from build123d import *

# Parameters (mm, degrees)
EXTRU_MINCE1_DEPTH    = 55
D_GAGEMENT_M41_D      = 4.5
D_GAGEMENT_M42_D      = 4.5
D_GAGEMENT_M271_D     = 30
D_GAGEMENT_M271_DEPTH = 1.5
D_GAGEMENT_M271_TIP   = 9.012909285


with BuildPart() as part:
    # Esquisse1 → Extru.-Mince1 (new body)
    with BuildSketch(Plane.XY):
        Polygon((0, 40), (0, 0), (25, 0), (25, 1.5), (1.5, 1.5), (1.5, 40), align=None)
    extrude(amount=-EXTRU_MINCE1_DEPTH)

    # Dégagement M41 (through all)
    with Locations(Plane(origin=(0, 1.5, 0), x_dir=(-1, 0, 0), z_dir=(0, 1, 0))):
        with Locations((-12.5, -7), (-12.5, -27.5), (-12.5, -48)):
            Hole(D_GAGEMENT_M41_D / 2)

    # Dégagement M42 (through all)
    with Locations(Plane(origin=(1.5, 0, 0), x_dir=(0, 0, -1), z_dir=(1, 0, 0))):
        with Locations((5, 34), (33, 6)):
            Hole(D_GAGEMENT_M42_D / 2)

    # Dégagement M271
    with Locations(Plane(origin=(1.5, 0, 0), x_dir=(0, 0, -1), z_dir=(1, 0, 0))):
        with Locations((19, 20)):
            Hole(D_GAGEMENT_M271_D / 2, depth=D_GAGEMENT_M271_DEPTH)
            with Locations((0, 0, -(D_GAGEMENT_M271_DEPTH + D_GAGEMENT_M271_TIP / 2))):  # 118° drill point
                Cone(0, D_GAGEMENT_M271_D / 2, D_GAGEMENT_M271_TIP, mode=Mode.SUBTRACT)


solid = part.part
Work out the finished part from the listing and answer in its coordinate system (mm). A direction names the side the tool comes from. Round coordinates to 2 decimals unless told otherwise and drop trailing zeros. Write each loop counter-clockwise with the first axis right and the second up, starting at its lowest first coordinate (ties: lowest second). Pieces come first, ordered by that corner, then holes.
1) The mould has two halves that part along Y. Classify faces 1 (the cylindrical face through (0.74, 6.676, -30.854)), 2 (the cylindrical face through (10.84, 0.74, -5.48)), 3 (the flat face through (10, 0, -27)): pulls with the +Y half, pulls with the -Y half, needs draft (parallel to the pull), parting line crosses it, or undercut.
2) A cutting plane is placed at B-B (z = -19). Give the vertices of the cut face in (x, y).
3) A cutting plane is placed at A-A (x = 12.5). Give the vertices of the cut face in (y, z), plus the area to 4 significant figures.
4) Straight lines are drawn through the part: line 1 (Z direction, x = 12.5, y = 0.35); line 2 (Z direction, x = 0.6, y = 20); line 3 (Y direction, x = 14.5, z = -37). For each, find the intervals that lie inside material, in ascending order.
5) A cutting plane is placed at D-D (z = -33). Give the vertices of the cut face in (x, y), plus the area to 3 significant figures.
6) Given pin 1 Ø1.5 at (x, z) = (11, -21) entering from -Y; pin 2 Ø11.5 at (y, z) = (12, -41) entering from +X, each flat-ended and moving along its own axis, determine where each tip first touches the part or whether it passes through.
7) A tool of negligible diameter and unlimited length cuts with its end or side. For faces 4 (the flat face through (16, 1.5, -27)), 5 (the cylindrical face through (0.74, 36.23, -5.29)), from which of +Z, -Z, +X, -X, +Y, -Y can it reach the whole face along a straight path? Write none if from no direction.
8) A cutting plane is placed at C-C (y = 34). Give the vertices of the cut face in (x, z).
Completed:
1. face 1: undercut
1. face 2: needs draft
1. face 3: pulls with the -Y half
2. outline: (0, 0) - (25, 0) - (25, 1.5) - (1.5, 1.5) - (1.5, 5) - (0, 5) - close; (0, 35) - (1.5, 35) - (1.5, 40) - (0, 40) - close
3. outline: (0, -55) - (1.5, -55) - (1.5, -50.25) - (0, -50.25) - close; (0, -45.75) - (1.5, -45.75) - (1.5, -29.75) - (0, -29.75) - close; (0, -25.25) - (1.5, -25.25) - (1.5, -9.25) - (0, -9.25) - close; (0, -4.75) - (1.5, -4.75) - (1.5, 0) - (0, 0) - close
3. area: 62.25 mm2
4. line 1: z = -55 to -50.25, -45.75 to -29.75, -25.25 to -9.25, -4.75 to 0
4. line 2: z = -55 to -34, -4 to 0
4. line 3: y = 0 to 1.5
5. outline: (0, 0) - (25, 0) - (25, 1.5) - (1.5, 1.5) - (1.5, 3.75) - (0, 3.75) - close; (0, 8.25) - (1.5, 8.25) - (1.5, 14.61) - (0, 14.61) - close; (0, 25.39) - (1.5, 25.39) - (1.5, 40) - (0, 40) - close
5. area: 72.3 mm2
6. pin 1: stops at y = 0
6. pin 2: stops at x = 1.5
7. face 4: +Z, -Z, +X, +Y
7. face 5: +X, -X
8. outline: (0, -55) - (1.5, -55) - (1.5, -24.39) - (0, -24.39) - close; (0, -13.61) - (1.5, -13.61) - (1.5, -7.25) - (0, -7.25) - close; (0, -2.75) - (1.5, -2.75) - (1.5, 0) - (0, 0) - close
